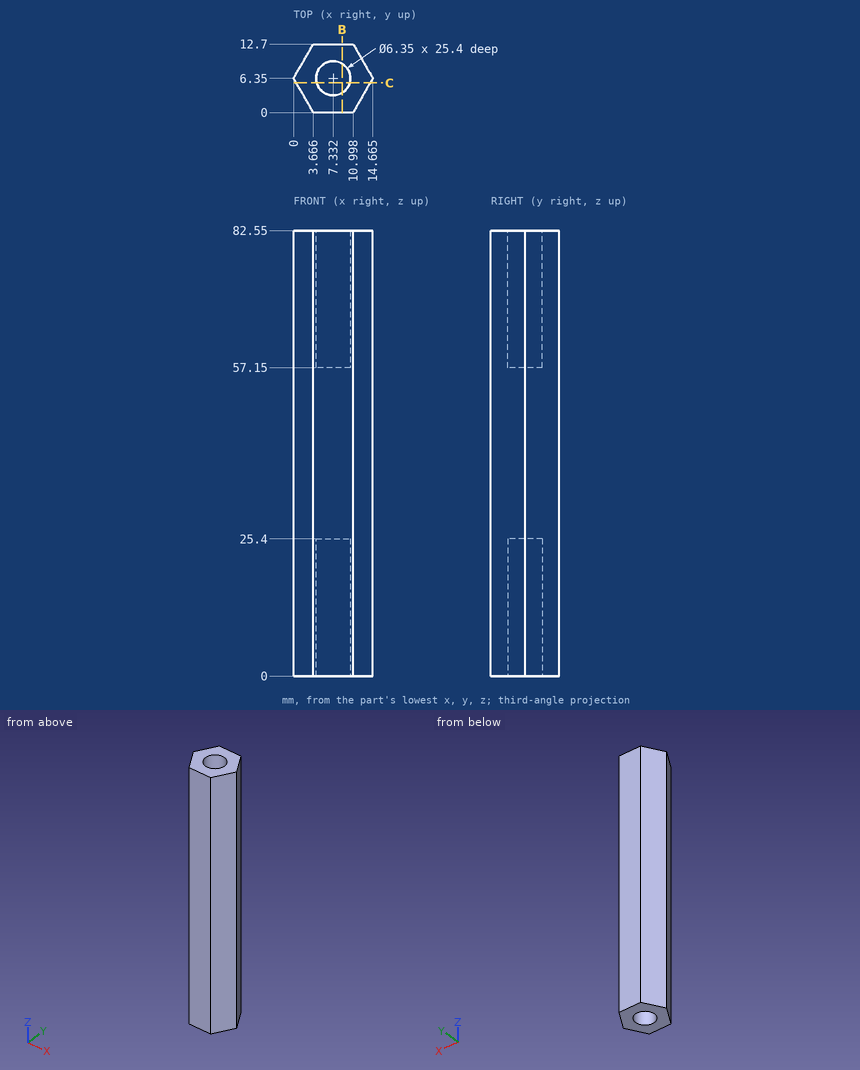
Input: dimensioned drawing with shaded views. Units: mm. Origin: part minimum x, y, z. Give positions to 0.01 mm unless a question says otherwise; leave off trailing zeros. Write each loop counter-clockwise with the first axis right and the second up, starting at its lowest first coordinate (ties: lowest second). Pieces come first, ordered by that corner, then holes. Notation, with made-up numbers: (69.25, 89) - (105.25, 89) arc R31 cw to (105.25, 122) - close; hole circle Ø10 at (56, 8.5). An arc over 180 degrees is marked (long way). Write item = value, one per line. Start each with the question number.
1) Material intervals for L1, parallel to Y at x = 7.25, z = 63.5 (1 decimal); L2, parallel to X at y = 5.5, z = 12.5 (1 decimal); L3, parallel to X at y = 6.5, z = 68 (1 decimal), sorted ascending. Write a range as [from, to].
2) Cut plane C-C (y = 5.5). Return loops of the section in (x, z).
3) Cut plane B-B (x = 9). Return loops of the section in (y, z).
4) Pin query (flat end, axial travel): pin 1 (2 mm diameter, centred on y = 2, z = 66.5, fed in from -X) (1 decimal); pin 2 (5 mm diameter, centred on x = 7.33, y = 6.35, fed in from -Z); pin 3 (5.5 mm diameter, centred on x = 7.33, y = 6.35, fed in from +Z). Return the tip coordinate at first contact, or that it passes through.
Answers follow:
q1.L1 = [0, 3.2], [9.5, 12.7]
q1.L2 = [0.5, 4.3], [10.4, 14.2]
q1.L3 = [0.1, 4.2], [10.5, 14.6]
q2.outline = (0.49, 0) - (4.27, 0) - (4.27, 25.4) - (10.39, 25.4) - (10.39, 0) - (14.17, 0) - (14.17, 82.55) - (10.39, 82.55) - (10.39, 57.15) - (4.27, 57.15) - (4.27, 82.55) - (0.49, 82.55) - close
q3.outline = (0, 0) - (3.65, 0) - (3.65, 25.4) - (9.05, 25.4) - (9.05, 0) - (12.7, 0) - (12.7, 82.55) - (9.05, 82.55) - (9.05, 57.15) - (3.65, 57.15) - (3.65, 82.55) - (0, 82.55) - close
q4.pin_1 = 1.9
q4.pin_2 = 25.4
q4.pin_3 = 57.15
